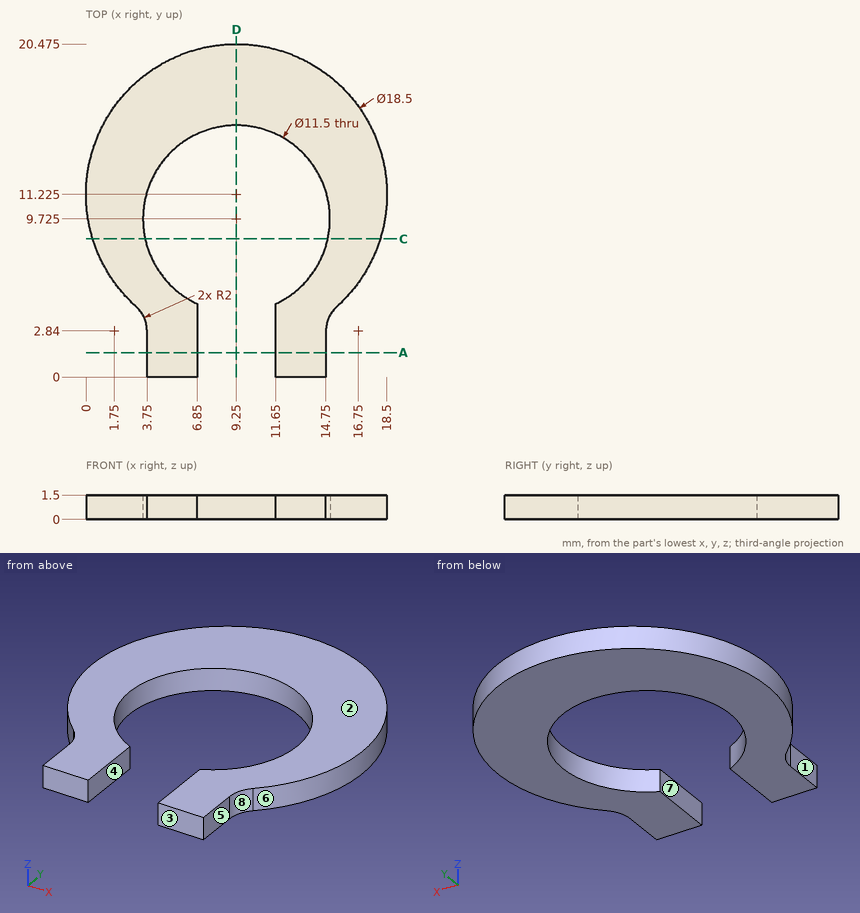
Source: three-view drawing plus pictorial views. Frame: mm from the lowest corner of the part. A direction names the side the tool comes from. Coordinates: 2 decimals unless noted, no trailing zeros. Loops run counter-clockwise (first coordinate to the right, second up) from the corner with the lowest first, then second, coordinate; pieces in that order, holes last. Notation, with made-up numbers: (10, 87.25) - (37, 87.25) arc R16 cw to (37, 95.25) - close; hole circle Ø2 at (-39, -30). An arc over 180 degrees is marked (long way). One line per item, written item: value. Start each with the question number.
1. Contact query for flat-ended pins moving along their axis: P1, Ø0.8, axis at y = 1, z = 0.5, coming from the -X side; P2, Ø7, axis at x = 9.25, y = 9.73, coming from the +Z side. Output: stop coordinate, or through.
2. Section A-A (y = 1.5). Return the cut outline in (x, z).
3. Ray query, L1, parallel to X at y = 2.75, z = 0.25; L2, parallel to Y at x = 9.25, z = 1.3 (1 decimal); L3, parallel to X at y = 9.5, z = 0.35. Return the intervals inside material, ascending.
4. Set-up query: the marked faces 1, 2, 3, 4 and 5. Return all of +Z, -Z, +X, -X, +Y, -Y with unobstructed straight access to the full face (end or side cutting, diameter ignored); none if empty.
5. Mould query, pull axis X, two halves, no side actions, for the marked faces 6, 7 and 8. Classes: pulls with the +X half, pulls with the -X half, needs draft (parallel to the pull), parting line crosses it, or undercut.
6. Section D-D (x = 9.25). Return the cut outline in (y, z) (1 decimal).
7. Section C-C (y = 8.5). Return the cut outline in (x, z).
Verdict:
1. P1: stops at x = 3.75
1. P2: passes through
2. outline: (3.75, 0) - (6.85, 0) - (6.85, 1.5) - (3.75, 1.5) - close; (11.65, 0) - (14.75, 0) - (14.75, 1.5) - (11.65, 1.5) - close
3. L1: x = 3.75 to 6.85, 11.65 to 14.75
3. L2: y = 15.5 to 20.5
3. L3: x = 0.16 to 3.5, 15 to 18.34
4. face 1: +Z, -Z, -X, -Y
4. face 2: +Z, +X, -X, +Y, -Y
4. face 3: +Z, -Z, +X, -X, -Y
4. face 4: +Z, -Z, -Y
4. face 5: +Z, -Z, +X, -Y
5. face 6: parting line crosses it
5. face 7: undercut
5. face 8: pulls with the +X half
6. outline: (15.5, 0) - (20.5, 0) - (20.5, 1.5) - (15.5, 1.5) - close
7. outline: (0.41, 0) - (3.63, 0) - (3.63, 1.5) - (0.41, 1.5) - close; (14.87, 0) - (18.09, 0) - (18.09, 1.5) - (14.87, 1.5) - close
